Work out the finished part from the listing and answer in its coordinate system (mm). A direction names the side the tool comes from. Round coordinates to 2 decimals unless told otherwise and drop trailing zeros. Write each loop counter-clockwise with the first axis right and the second up, starting at its lowest first coordinate (ties: lowest second). Pieces come first, ordered by that corner, then holes.
1. Find section D-D (x = 4). Write down the section's boundary in (y, z), and give its area (3 significant figures).
2. Straight lines are drawn through the part: probe 1 along Y at (x, z) = (0, 1.55); probe 2 along Y at (x, z) = (0, 4.1); probe 3 along Y at (x, z) = (25, 1.8). For each, find the intervals that lie inside material, in ascending order.
3. Find section A-A (z = 0.7). Count the separate pieces of the cut face and the enclosed holes in it, and give its area (3 significant figures).
4. Determine the mould class of faces 4 (the face through (-3, 19, 1)), 5 (the face through (0, 24, 2)), 6 (the face through (19, 3, 1)), 7 (the face through (-26, 0, 2)) for opening direction Y: pulls with the +Y half, pulls with the -Y half, needs draft (parallel to the pull), parting line crosses it, or undercut.
5. Flat-ended cylindrical pins translate along their axes: pin 1 Ø3.5 at (y, z) = (-21.5, 1) entering from -X; pin 2 Ø2.5 at (x, y) = (-25, 0) entering from +Z; pin 3 Ø0.9 at (x, z) = (-21.5, 2) entering from -Y. Find the tip coordinate at first contact, or state that the pin passes through.
6. Find section C-C (y = -6). Write down the section's boundary in (x, z).
7. A tool of negligible diameter and unlimited length cuts with its end or side. For faces 1 (the face through (19, -3, 1)), 2 (the face through (-19, 3, 1)), 3 (the face through (-19, -3, 1)), from which of +Z, -Z, +X, -X, +Y, -Y can it reach the whole face along a straight path? Write none if from no direction.
8. Find section B-B (z = 4.5). Write down the section's boundary in (x, y).
```python
from build123d import *

# Parameters (mm, degrees)
SKETCH1_R           = 0.8
BOSS_EXTRUDE1_DEPTH = 3
FILLET1_R           = 10
SKETCH2_R           = 2
CUT_EXTRUDE1_DEPTH  = 3
SKETCH3_R           = 8
SKETCH3_R_2         = 2
SKETCH3_R_3         = 0.8
BOSS_EXTRUDE2_DEPTH = 3
SKETCH4_R           = 1
CUT_EXTRUDE2_DEPTH  = 3


with BuildPart() as part:
    # Sketch1 → Boss-Extrude1 (new body)
    # profile 1 of 2: a face of its own
    with BuildSketch(Plane.XY):
        with BuildLine():
            Line((25, -3), (-25, -3))
            ThreePointArc((-25, -3), (-28, 0), (-25, 3))
            Line((-25, 3), (25, 3))
            ThreePointArc((25, 3), (28, 0), (25, -3))
        make_face()
        with Locations((-6, 0)):
            Circle(SKETCH1_R, mode=Mode.SUBTRACT)
        with Locations((6, 0)):
            Circle(SKETCH1_R, mode=Mode.SUBTRACT)
    # profile 2 of 2: a face of its own
    with BuildSketch(Plane.XY):
        with BuildLine():
            Line((-3, -25), (-3, 25))
            ThreePointArc((-3, 25), (0, 28), (3, 25))
            Line((3, 25), (3, -25))
            ThreePointArc((3, -25), (0, -28), (-3, -25))
        make_face()
        with Locations((0, 6)):
            Circle(SKETCH1_R, mode=Mode.SUBTRACT)
        with Locations((0, -6)):
            Circle(SKETCH1_R, mode=Mode.SUBTRACT)
    extrude(amount=BOSS_EXTRUDE1_DEPTH)

    # Fillet1
    fillet1_edges = [part.edges().sort_by_distance(p)[0] for p in [
        (3, -3, 1.5),
        (-3, -3, 1.5),
        (-3, 3, 1.5),
        (3, 3, 1.5),
    ]]
    fillet(fillet1_edges, radius=FILLET1_R)

    # Sketch2 → Cut-Extrude1 (cut)
    with BuildSketch(Plane.XY.offset(3)):
        Circle(SKETCH2_R)
    extrude(amount=-CUT_EXTRUDE1_DEPTH, mode=Mode.SUBTRACT)

    # Sketch3 → Boss-Extrude2 (add)
    with BuildSketch(Plane.XY.offset(3)):
        Circle(SKETCH3_R)
        Circle(SKETCH3_R_2, mode=Mode.SUBTRACT)
        with Locations((0, 6)):
            Circle(SKETCH3_R_3, mode=Mode.SUBTRACT)
        with Locations((6, 0)):
            Circle(SKETCH3_R_3, mode=Mode.SUBTRACT)
        with Locations((0, -6)):
            Circle(SKETCH3_R_3, mode=Mode.SUBTRACT)
        with Locations((-6, 0)):
            Circle(SKETCH3_R_3, mode=Mode.SUBTRACT)
    extrude(amount=BOSS_EXTRUDE2_DEPTH)

    # Sketch4 → Cut-Extrude2 (cut)
    with BuildSketch(Plane.XY.offset(3)):
        with Locations((0, 25)):
            Circle(SKETCH4_R)
        with Locations((25, 0)):
            Circle(SKETCH4_R)
        with Locations((0, -25)):
            Circle(SKETCH4_R)
        with Locations((-25, 0)):
            Circle(SKETCH4_R)
    extrude(amount=-CUT_EXTRUDE2_DEPTH, mode=Mode.SUBTRACT)


solid = part.part
```
Worked answers:
1. outline: (-8.64, 0) - (8.64, 0) - (8.64, 3) - (6.93, 3) - (6.93, 6) - (-6.93, 6) - (-6.93, 3) - (-8.64, 3) - close
1. area: 93.4 mm2
2. probe 1: y = -28 to -26, -24 to -6.8, -5.2 to -2, 2 to 5.2, 6.8 to 24, 26 to 28
2. probe 2: y = -8 to -6.8, -5.2 to -2, 2 to 5.2, 6.8 to 8
2. probe 3: y = -3 to -1, 1 to 3
3. separate pieces: 1
3. enclosed holes: 9
3. area: 673 mm2
4. face 4: needs draft
4. face 5: undercut
4. face 6: pulls with the +Y half
4. face 7: undercut
5. pin 1: stops at x = -3
5. pin 2: stops at z = 3
5. pin 3: stops at y = -3
6. outline: (-5.86, 0) - (-0.8, 0) - (-0.8, 6) - (-5.29, 6) - (-5.29, 3) - (-5.86, 3) - close; (0.8, 0) - (5.86, 0) - (5.86, 3) - (5.29, 3) - (5.29, 6) - (0.8, 6) - close
7. face 1: +Z, -Z, +X, -Y
7. face 2: +Z, -Z, -X, +Y
7. face 3: +Z, -Z, -X, -Y
8. outline: circle Ø16 at (0, 0); hole circle Ø1.6 at (-6, 0); hole circle Ø4 at (0, 0); hole circle Ø1.6 at (0, -6); hole circle Ø1.6 at (0, 6); hole circle Ø1.6 at (6, 0)
